from build123d import *

# Parameters (mm, degrees)
F0_R     = 19.05
F1_DEPTH = 38.1
F2_DEPTH = 31.75
F0_R_2   = 6.35
F3_DEPTH = 25.4


with BuildPart() as f1:
    # F0 (on Top) → F1 (new body)
    with BuildSketch(Plane.XY):
        with BuildLine():
            Line((-84.90175, 24.89703), (-89.931453, 25.4))
            ThreePointArc((-89.931453, 25.4), (-115.331453, 0), (-89.931453, -25.4))
            Line((-89.931453, -25.4), (-84.90175, -24.89703))
            ThreePointArc((-84.90175, -24.89703), (-70.272937, -16.08424), (-64.531453, 0))
            ThreePointArc((-64.531453, 0), (-70.272937, 16.08424), (-84.90175, 24.89703))
        make_face()
        with Locations((-89.931453, 0)):
            Circle(F0_R, mode=Mode.SUBTRACT)
    extrude(amount=F1_DEPTH)

    # F0 (on Top) → F2 (join)
    with BuildSketch(Plane.XY):
        with Locations((-89.931453, 0)):
            Circle(F0_R)
    extrude(amount=F2_DEPTH)

    # F0 (on Top) → F3 (join)
    with BuildSketch(Plane.XY):
        with BuildLine():
            Line((-84.90175, 24.89703), (-89.931453, 25.4))
            ThreePointArc((-89.931453, 25.4), (-115.331453, 0), (-89.931453, -25.4))
            Line((-89.931453, -25.4), (-84.90175, -24.89703))
            ThreePointArc((-84.90175, -24.89703), (-70.272937, -16.08424), (-64.531453, 0))
            ThreePointArc((-64.531453, 0), (-70.272937, 16.08424), (-84.90175, 24.89703))
        make_face()
        with Locations((-89.931453, 0)):
            Circle(F0_R, mode=Mode.SUBTRACT)
        with BuildLine():
            ThreePointArc((-84.90175, 24.89703), (-87.404058, 25.273945), (-89.931453, 25.4))
            Line((-89.931453, 25.4), (-84.90175, 24.89703))
        make_face()
        with BuildLine():
            Line((-84.90175, -24.89703), (-89.931453, -25.4))
            ThreePointArc((-89.931453, -25.4), (-87.404058, -25.273945), (-84.90175, -24.89703))
        make_face()
        with BuildLine():
            Line((37.068547, 12.7), (-84.90175, 24.89703))
            ThreePointArc((-84.90175, 24.89703), (-70.272937, 16.08424), (-64.531453, 0))
            ThreePointArc((-64.531453, 0), (-70.272937, -16.08424), (-84.90175, -24.89703))
            Line((-84.90175, -24.89703), (37.068547, -12.7))
            ThreePointArc((37.068547, -12.7), (24.368547, 0), (37.068547, 12.7))
        make_face()
        with BuildLine():
            ThreePointArc((-51.831453, -6.35), (-58.181453, 0), (-51.831453, 6.35))
            Line((-51.831453, 6.35), (-1.031453, 6.35))
            ThreePointArc((-1.031453, 6.35), (5.318547, 0), (-1.031453, -6.35))
            Line((-1.031453, -6.35), (-51.831453, -6.35))
        make_face(mode=Mode.SUBTRACT)
        with BuildLine():
            ThreePointArc((49.768547, 0), (46.048803, 8.980256), (37.068547, 12.7))
            ThreePointArc((37.068547, 12.7), (24.368547, 0), (37.068547, -12.7))
            ThreePointArc((37.068547, -12.7), (46.048803, -8.980256), (49.768547, 0))
        make_face()
        with Locations((37.068547, 0)):
            Circle(F0_R_2, mode=Mode.SUBTRACT)
    extrude(amount=F3_DEPTH)


solid = f1.part
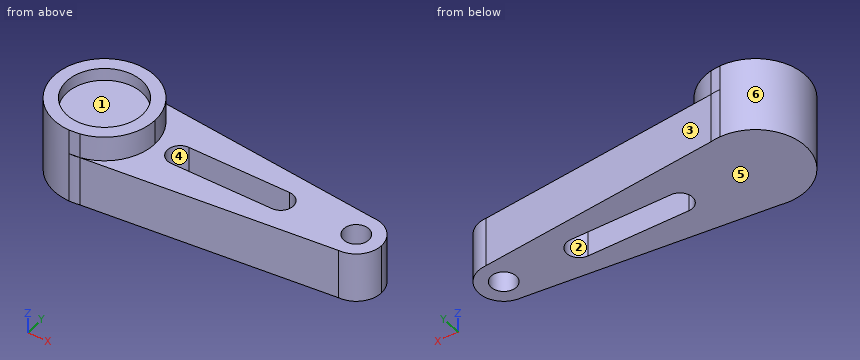
The model under review builds one solid part; all positions refer to its coordinate system, in mm. Face numbers are marked on the shaded views. A direction names the side the tool comes from. Round coordinates to 2 decimals unless told otherwise and drop trailing zeros. Order: outer loops, then holes, each group sorted by start corner. A loop starts at its lowest first (then second) coordinate and runs counter-clockwise, first axis right, second up. Notation, with made-up numbers: (76.5, -1.5) -> (100.5, -1.5) arc R23 ccw to (100.5, 12.5) -> close; hole circle Ø1 at (-35, -10.75). An arc over 180 degrees is marked (long way). Return JSON: item names as keys, results as strings.
1. Take a section at C-C (z = 34). Write out the cut boundary in (x, y).
Answer block:
{"outline": "(-89.93, -25.4) -> (-84.9, -24.9) arc R25.4 ccw to (-64.53, 0) arc R25.4 ccw to (-84.9, 24.9) -> (-89.93, 25.4) arc R25.4 ccw to start; hole circle Ø38.1 at (-89.93, 0)"}
2. Take a section at B-B (x = -32). Write out the cut boundary in (y, z).
Answer block:
{"outline": "(-19.61, 0) -> (-6.35, 0) -> (-6.35, 25.4) -> (-19.61, 25.4) -> close; (6.35, 0) -> (19.61, 0) -> (19.61, 25.4) -> (6.35, 25.4) -> close"}
3. For the marked faces 1, 2 and 3, list the 3-axis set-ups (+Z, -Z, +X, -X, +Y, -Y) from which the entire face can be reached by the end or side of a thin tool; tool diameter is ignored.
Answer block:
{"face 1": "+Z", "face 2": "+Z, -Z", "face 3": "+Z, -Z, +X, +Y"}
4. For L1, parallel to X at y = -2.5, z = 9; L2, parallel to Y at x = -91, z = 33; L3, parallel to Z at x = -47, y = 15.5, list the stretches that pass through material, from the lowest coordinate up. Write a range as [from, to].
Answer block:
{"L1": "x = [-115.21, -57.67], [4.81, 31.23], [42.91, 49.52]", "L2": "y = [-25.38, -19.02], [19.02, 25.38]", "L3": "z = [0, 25.4]"}
5. Take a section at D-D (y = -4). Write out the cut boundary in (x, z), then the cut area to 3 significant figures.
Answer block:
{"outline": "(-115.01, 0) -> (-56.76, 0) -> (-56.76, 25.4) -> (-64.85, 25.4) -> (-64.85, 38.1) -> (-71.31, 38.1) -> (-71.31, 31.75) -> (-108.56, 31.75) -> (-108.56, 38.1) -> (-115.01, 38.1) -> close; (3.9, 0) -> (32.14, 0) -> (32.14, 25.4) -> (3.9, 25.4) -> close; (42, 0) -> (49.12, 0) -> (49.12, 25.4) -> (42, 25.4) -> close", "area": "2,780 mm²"}
6. Insertion check: P1, Ø11.5, axis at x = -95.5, y = 3.5, coming from the +Z side; P2, Ø20.5, axis at x = -22, z = 8.5, coming from the -Y side; P3, Ø25, axis at x = -43.5, y = -3, coming from the +Z side; P4, Ø11.5, axis at x = 37.07, y = 0, coming from the +Z side. Each pin has a flat end and moves straight along its axis. Give the tip position at first contact, or say it passes through.
Answer block:
{"P1": "stops at z = 31.75", "P2": "stops at y = -19.63", "P3": "stops at z = 25.4", "P4": "passes through"}
7. The part is to be moulded in two halves that separate along X. For the marked faces 4, 5 and 6, say which applies: +X half, -X half, draft (parallel to the pull), parting line (faces both ways), or undercut.
Answer block:
{"face 4": "undercut", "face 5": "draft", "face 6": "-X half"}
8. Take a section at A-A (z = 11.5). Write out the cut boundary in (x, y), then the cut area to 3 significant figures.
Answer block:
{"outline": "(-89.93, -25.4) arc R25.4 ccw to (-84.9, -24.9) -> (37.07, -12.7) arc R12.7 ccw to (37.07, 12.7) -> (-84.9, 24.9) arc R25.4 ccw to (-89.93, 25.4) arc R25.4 ccw to start; hole (-51.83, -6.35) -> (-1.03, -6.35) arc R6.35 ccw to (-1.03, 6.35) -> (-51.83, 6.35) arc R6.35 ccw to start; hole circle Ø12.7 at (37.07, 0)", "area": "5,210 mm²"}
